Here's how the part is built. I have some questions about the finished solid (model axes, mm). Round coordinates to 2 decimals unless told otherwise and drop trailing zeros. Write each loop counter-clockwise with the first axis right and the second up, starting at its lowest first coordinate (ties: lowest second). Pieces come first, ordered by that corner, then holes. Notation, with made-up numbers: M 44.25,42 L 98.25,42 A35 ccw 98.25,75 Z; hole C -32.75,-30 d3. An arc over 180 degrees is marked long. Write item = value, one per line. Start each with the question number.
(1) I want a section at B-B (x = -10). List the corners of the cut face in (y, z) for me.
(2) I want a section at C-C (z = 0.75). Give the number of separate pieces and of enclosed holes in the cut face, and give its area (3 significant figures).
(3) If we mould it in two halves opening along X, with no side actions, what happens to faces 1 (the flat face through (-27.5, 0, 1)), 2 (the cylindrical face through (25.219, 25.095, 1.521)), 3 (the cylindrical face through (12.89, -22.51, 1.48))? For each: released by +X, released by -X, zero draft, split by the parting line, or undercut.
(4) Will this pin go through, and if not, where does the flat tip stop? pin 1 Ø2.5 at (x, y) = (16, -13.5) entering from -Z.
(5) I want a section at D-D (y = -21.5). List the corners of the cut face in (x, z) for me.
(6) I want a section at A-A (y = -13.5). List the corners of the cut face in (x, z) for me.
(7) I need wall thicknesses on line 1 along Y through (x, z) = (-16, 0.7); line 2 along Y through (x, z) = (17, 2.6); line 3 along X through (y, z) = (-21, 1.6). Which ranges of each line are inside material? Lowest first, please.
Autodesk Inventor part; units mm, degrees
ref_plane "YZ Plane" through (0, 0, 0) normal (1, 0, 0) x (0, 1, 0)
ref_plane "XZ Plane" through (0, 0, 0) normal (0, 1, 0) x (-1, 0, 0)
ref_plane "XY Plane" through (0, 0, 0) normal (0, 0, 1) x (1, 0, 0)
sketch "Sketch1" plane through (0, 0, 0) normal (0, 0, 1) x (1, 0, 0)
  point P0 (0, 0)
sketch "Sketch2" plane through (0, 0, 0) normal (0, 0, 1) x (1, 0, 0)
  line L0 (27.5, -27.5002) -> (-27.5, -27.5002)
  line L1 (-27.5, -27.5002) -> (-27.5, 27.5002)
  line L2 (-27.5, 27.5002) -> (27.5, 27.5002)
  line L3 (27.5, 27.5002) -> (27.5, -27.5002)
  circle A0 centre (16, 13.5) radius 1.5
  circle A1 centre (-16, 13.5) radius 1.5
  circle A2 centre (-16, -13.5) radius 1.5
  circle A3 centre (16, -13.5) radius 1.5
  circle A4 centre (14, -21.5) radius 1.5
  circle A5 centre (-14, -21.5) radius 1.5
  circle A6 centre (10, 21.5) radius 1.2498
  circle A7 centre (-10, 21.5) radius 1.2498
extrude "Extrusion3" add sketch "Sketch2" along normal blind 3
fillet "Fillet3" radius 8 4 edges at (27.5, 27.5002, 1.5) (-27.5, 27.5002, 1.5) (27.5, -27.5002, 1.5) (-27.5, -27.5002, 1.5)
properties part number "retractable_landing_skids_adapter_plate" material "CFRP"
Returned:
q1.outline = M -27.5,0 L 20.25,0 L 20.25,3 L -27.5,3 Z; M 22.75,0 L 27.5,0 L 27.5,3 L 22.75,3 Z
q2.separate_pieces = 1
q2.enclosed_holes = 8
q2.area = 2,920 mm²
q3.face_1 = released by -X
q3.face_2 = released by +X
q3.face_3 = undercut
q4.pin_1 = through
q5.outline = M -27.25,0 L -15.5,0 L -15.5,3 L -27.25,3 Z; M -12.5,0 L 12.5,0 L 12.5,3 L -12.5,3 Z; M 15.5,0 L 27.25,0 L 27.25,3 L 15.5,3 Z
q6.outline = M -27.5,0 L -17.5,0 L -17.5,3 L -27.5,3 Z; M -14.5,0 L 14.5,0 L 14.5,3 L -14.5,3 Z; M 17.5,0 L 27.5,0 L 27.5,3 L 17.5,3 Z
q7.line_1 = -27.5 to -15, -12 to 12, 15 to 27.5
q7.line_2 = -27.5 to -14.62, -12.38 to 12.38, 14.62 to 27.5
q7.line_3 = -27.36 to -15.41, -12.59 to 12.59, 15.41 to 27.36
